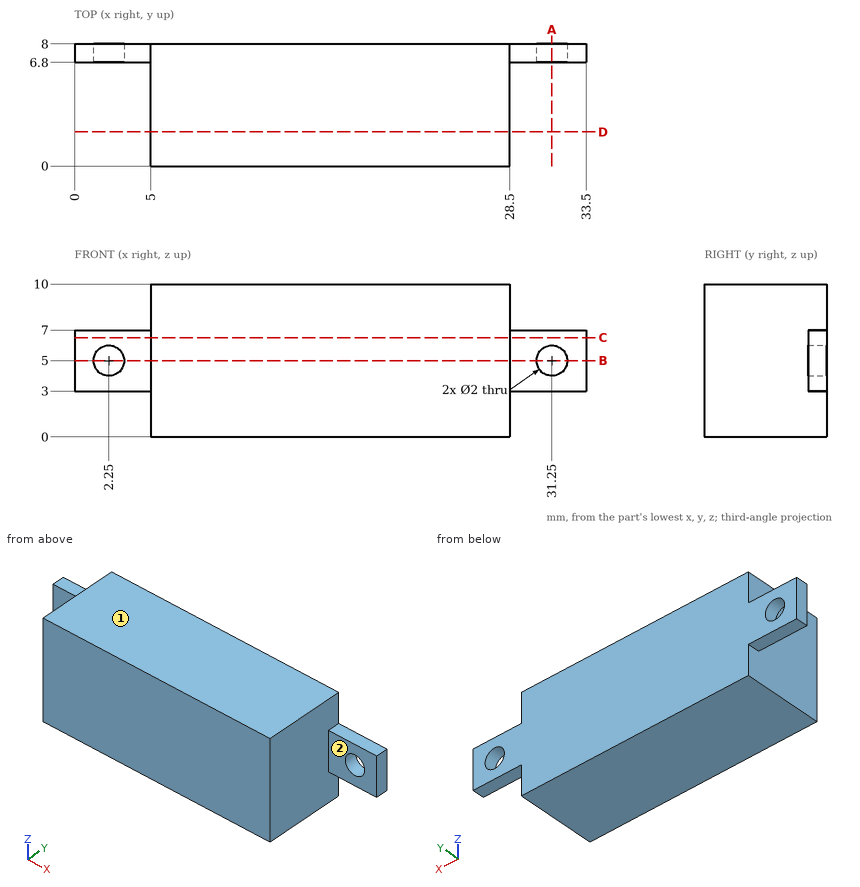
Source: three-view drawing plus pictorial views. Frame: mm from the lowest corner of the part. A direction names the side the tool comes from. Coordinates: 2 decimals unless noted, no trailing zeros. Order: outer loops, then holes, each group sorted by start corner. A loop starts at its lowest first (then second) coordinate and runs counter-clockwise, first axis right, second up. Notation, with made-up numbers: M 49.25,71 L 81.25,71 A24 ccw 81.25,86 Z; hole C -33,24.25 d10. An arc over 180 degrees is marked long. Write each question's results on one line, items separated by ' | '. Start each with the question number.
1. Section D-D, the plane y = 2.25. Return the cut outline in (x, z).
2. Material intervals for L1, parallel to X at y = 7.3, z = 5; L2, parallel to X at y = 7, z = 2.25; L3, parallel to Y at x = 1, z = 6.5, sorted ascending.
3. Section B-B, the plane z = 5. Return the cut outline in (x, y).
4. Reachability of the marked faces 1 and 2 from +Z, -Z, +X, -X, +Y, -Y: full face, straight path, thin tool, end or side. Return the list, or none.
5. Pin query (flat end, axial travel): pin 1 (2 mm diameter, centred on y = 6.5, z = 2, fed in from +X); pin 2 (1.2 mm diameter, centred on x = 2.25, z = 5, fed in from -Y); pin 3 (1 mm diameter, centred on x = 31.5, y = 7, fed in from +Z); pin 4 (1 mm diameter, centred on y = 5.5, z = 1.5, fed in from -X). Return the tip coordinate at first contact, or that it passes through.
6. Section A-A, the plane x = 31.25. Return the cut outline in (y, z).
7. Section C-C, the plane z = 6.5. Return the cut outline in (x, y), then the cut area to 3 significant figures.
Solution:
1) outline: M 5,0 L 28.5,0 L 28.5,10 L 5,10 Z
2) L1: 0 to 1.25, 3.25 to 30.25, 32.25 to 33.5 | L2: 5 to 28.5 | L3: 6.8 to 8
3) outline: M 0,6.8 L 1.25,6.8 L 1.25,8 L 0,8 Z; M 3.25,6.8 L 5,6.8 L 5,0 L 28.5,0 L 28.5,6.8 L 30.25,6.8 L 30.25,8 L 3.25,8 Z; M 32.25,6.8 L 33.5,6.8 L 33.5,8 L 32.25,8 Z
4) face 1: +Z, +X, -X, +Y, -Y | face 2: +Z, -Z, +X, -Y
5) pin 1: x = 28.5 | pin 2: through | pin 3: z = 7 | pin 4: x = 5
6) outline: M 6.8,3 L 8,3 L 8,4 L 6.8,4 Z; M 6.8,6 L 8,6 L 8,7 L 6.8,7 Z
7) outline: M 0,6.8 L 5,6.8 L 5,0 L 28.5,0 L 28.5,6.8 L 33.5,6.8 L 33.5,8 L 0,8 Z | area: 200 mm²
